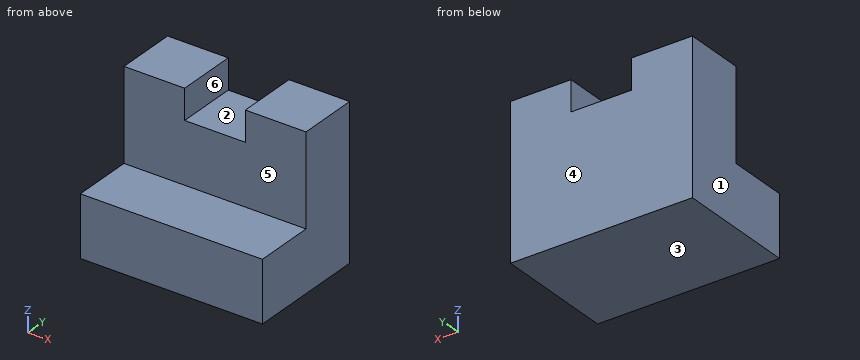
from build123d import *

# Parameters (mm, degrees)
F1_DEPTH = 38.1
F2_W     = 12.7
F2_H     = 6.35
F3_DEPTH = 81
F4_W     = 12.7
F4_H     = 6.35
F5_DEPTH = 81
F6_W     = 12.7
F6_H     = 6.35
F7_DEPTH = 81
F8_DEPTH = 25.401


# Not quite as in the source:
# - an extrude ends at something that could not be found from the text; its depth is read off the source's solid


with BuildPart() as f1:
    # F0 (on Right) → F1 (new body)
    with BuildSketch(Plane.YZ):
        Polygon((0, 0), (0, 31.75), (-12.7, 31.75), (-12.7, 12.7), (-25.4, 12.7), (-25.4, 0), align=None)
    extrude(amount=F1_DEPTH)

    # F2 (on Front) → F3 (cut, through all)
    with BuildSketch(Plane.XZ):
        with Locations((19.05, 29.0438578556)):
            Rectangle(F2_W, F2_H)
    extrude(amount=-F3_DEPTH, mode=Mode.SUBTRACT)

    # F4 (on Front) → F5 (cut, through all)
    with BuildSketch(Plane.XZ):
        with Locations((19.05, 28.5938853313)):
            Rectangle(F4_W, F4_H)
    extrude(amount=-F5_DEPTH, mode=Mode.SUBTRACT)

    # F6 (on Front) → F7 (cut, through all)
    with BuildSketch(Plane.XZ):
        with Locations((19.05, 28.9610116338)):
            Rectangle(F6_W, F6_H)
    extrude(amount=-F7_DEPTH, mode=Mode.SUBTRACT)

    # F4 (on Front) → F8 (cut, through all)
    with BuildSketch(Plane.XZ):
        with Locations((19.05, 28.5938853313)):
            Rectangle(F4_W, F4_H)
    extrude(amount=F8_DEPTH, mode=Mode.SUBTRACT)


solid = f1.part
Source: CAD feature listing. Evaluate the final solid. Frame: model axes, mm. Face numbers are marked on the shaded views. A direction names the side the tool comes from. Coordinates: 2 decimals unless noted, no trailing zeros. Loops run counter-clockwise (first coordinate to the right, second up) from the corner with the lowest first, then second, coordinate; pieces in that order, holes last. Notation, with made-up numbers: (1.25, 37.5) - (52.25, 37.5) arc R23 cw to (52.25, 66.5) - close; hole circle Ø6 at (25, 19). An arc over 180 degrees is marked (long way). One line per item, written item: value. Start each with the question number.
1. Set-up query: the marked faces 4, 5 and 6. Return all of +Z, -Z, +X, -X, +Y, -Y with unobstructed straight access to the full face (end or side cutting, diameter ignored); none if empty.
2. Ray query, L1, parallel to Z at x = 23.5, y = -10.25; L2, parallel to Z at x = 21, y = -17.5; L3, parallel to Y at x = 35, z = 17. Return the intervals inside material, ascending.
3. Mould query, pull axis X, two halves, no side actions, for the marked faces 1, 2 and 3. Classes: pulls with the +X half, pulls with the -X half, needs draft (parallel to the pull), parting line crosses it, or undercut.
4. Section B-B (y = -9). Return the cut outline in (x, z).
5. Contact query for flat-ended pins moving along their axis: P1, Ø10, axis at x = 11.5, y = -22.5, coming from the +Z side; P2, Ø1, axis at x = 31, z = 18.5, coming from the -Y side. Output: stop coordinate, or through.
6. Section C-C (x = 11.5). Return the cut outline in (y, z).
7. Section A-A (z = 26). Return the cut outline in (x, y).
8. Section D-D (z = 15). Return the cut outline in (x, y), and give its area (3 significant figures).
Verdict:
1. face 4: +Z, -Z, +X, -X, +Y
1. face 5: +Z, +X, -X, -Y
1. face 6: +Z, +Y, -Y
2. L1: z = 0 to 25.42
2. L2: z = 0 to 12.7
2. L3: y = -12.7 to 0
3. face 1: pulls with the -X half
3. face 2: undercut
3. face 3: needs draft
4. outline: (0, 0) - (38.1, 0) - (38.1, 31.75) - (25.4, 31.75) - (25.4, 25.42) - (12.7, 25.42) - (12.7, 31.75) - (0, 31.75) - close
5. P1: stops at z = 12.7
5. P2: stops at y = -12.7
6. outline: (-25.4, 0) - (0, 0) - (0, 31.75) - (-12.7, 31.75) - (-12.7, 12.7) - (-25.4, 12.7) - close
7. outline: (0, -12.7) - (12.7, -12.7) - (12.7, 0) - (0, 0) - close; (25.4, -12.7) - (38.1, -12.7) - (38.1, 0) - (25.4, 0) - close
8. outline: (0, -12.7) - (38.1, -12.7) - (38.1, 0) - (0, 0) - close
8. area: 484 mm2
